from build123d import *

# Parameters (mm, degrees)
SKETCH1_W                  = 5
SKETCH1_H                  = 7
BOSS_EXTRUDE1_DEPTH        = 2.5
SKETCH2_R                  = 0.75
CUT_EXTRUDE1_DEPTH         = 6.5
SKETCH4_R                  = 0.375
CHAMFER1_SIZE              = 0.1
SKETCH5_W                  = 0.8
SKETCH5_H                  = 0.1
CUT_EXTRUDE2_DEPTH         = 10.09068901
LPATTERN1_COUNT            = 2
LPATTERN1_PITCH            = 2.5
LPATTERN2_COUNT            = 2
LPATTERN2_PITCH            = 2.5
CHAMFER1_OF_LPATTERN2_SIZE = 0.1


with BuildPart() as part:
    # Sketch1 → Boss-Extrude1 (new body)
    with BuildSketch(Plane(origin=(0, 0, 0), x_dir=(1, 0, 0), z_dir=(0, 1, 0))):
        Rectangle(SKETCH1_W, SKETCH1_H)
    extrude(amount=BOSS_EXTRUDE1_DEPTH)

    # Sketch2 → Cut-Extrude1 (cut)
    with BuildSketch(Plane(origin=(0, 0, -3.5), x_dir=(-1, 0, 0), z_dir=(0, 0, -1))):
        with Locations((-1.2, 1.25)):
            Circle(SKETCH2_R)
    cut_extrude1 = extrude(amount=-CUT_EXTRUDE1_DEPTH, mode=Mode.SUBTRACT)

    # Sweep1: sweep along a path in Sketch3
    with BuildLine(Plane(origin=(1.2, 0, 0), x_dir=(0, 0, -1), z_dir=(1, 0, 0))) as sweep1_path:
        Line((-3.5, 1.254208417), (-3.8, 1.254208417))
        ThreePointArc((-3.8, 1.254208417), (-4.294974747, 1.049183164), (-4.5, 0.554208417))
        Line((-4.5, 0.554208417), (-4.5, -0.992950224))
    # Sketch4 → Sweep1 (sweep)
    with BuildSketch(Plane.XY.offset(3.5)):
        with Locations((1.2, 1.254208417)):
            Circle(SKETCH4_R)
    sweep1 = sweep(path=sweep1_path.line)

    # Chamfer1
    chamfer1_edges = [part.edges().sort_by_distance(p)[0] for p in [
        (0.825, 1.254208417, 3.5),
        (0.825, -0.992950224, 4.5),
    ]]
    chamfer(chamfer1_edges, length=CHAMFER1_SIZE)

    # Sketch5 → Cut-Extrude2 (cut, through all)
    with BuildSketch(Plane(origin=(0, 0, -3.5), x_dir=(-1, 0, 0), z_dir=(0, 0, -1))):
        with Locations((0, 2.45)):
            Rectangle(SKETCH5_W, SKETCH5_H)
    cut_extrude2 = extrude(amount=-CUT_EXTRUDE2_DEPTH, mode=Mode.SUBTRACT)

    # Mirror6: Cut-Extrude2 across plane
    add(cut_extrude2.mirror(Plane(origin=(0, 1.25, 0), x_dir=(0, 0, 1), z_dir=(0, -1, 0))), mode=Mode.SUBTRACT)

    # LPattern1: Cut-Extrude1 ×2
    with Locations(*[(-i * LPATTERN1_PITCH, 0, 0) for i in range(1, LPATTERN1_COUNT)]):
        add(cut_extrude1, mode=Mode.SUBTRACT)

    # LPattern2: Sweep1 ×2
    with Locations(*[(-i * LPATTERN2_PITCH, 0, 0) for i in range(1, LPATTERN2_COUNT)]):
        add(sweep1)

    # Chamfer1 of LPattern2
    chamfer1_of_lpattern2_edges = [part.edges().sort_by_distance(p)[0] for p in [
        (-1.675, 1.254208417, 3.5),
        (-1.675, -0.992950224, 4.5),
    ]]
    chamfer(chamfer1_of_lpattern2_edges, length=CHAMFER1_OF_LPATTERN2_SIZE)


solid = part.part
Here's how the part is built. I have some questions about the finished solid (model axes, mm). A direction names the side the tool comes from. Round coordinates to 2 decimals unless told otherwise and drop trailing zeros. Loops run counter-clockwise (first coordinate to the right, second up) from the corner with the lowest first, then second, coordinate; pieces in that order, holes last.
1. We'd pull the mould along X, two halves only. Please class faces 4 (the face through (2.5, 1, 0)), 5 (the face through (-1, 2.5, 0)), 6 (the face through (1, 1, 3)): +X half, -X half, draft (parallel to the pull), parting line (faces both ways), or undercut.
Answer list:
face 4: +X half
face 5: draft
face 6: undercut
2. If we section it at A-A on y = 0.4: Write out the boundary of the cut face in (x, z) (3 decimals).
Answer list:
outline: (-2.5, -3.5) - (2.5, -3.5) - (2.5, 3.5) - (-2.5, 3.5) - close; circle Ø0.75 at (-1.3, 4.5); circle Ø0.75 at (1.2, 4.5)
3. If we section it at B-B on z = -0.25: Write out the boundary of the cut face in (x, y).
Answer list:
outline: (-2.5, 0) - (-0.4, 0) - (-0.4, 0.1) - (0.4, 0.1) - (0.4, 0) - (2.5, 0) - (2.5, 2.5) - (0.4, 2.5) - (0.4, 2.4) - (-0.4, 2.4) - (-0.4, 2.5) - (-2.5, 2.5) - close; hole circle Ø1.5 at (-1.3, 1.25); hole circle Ø1.5 at (1.2, 1.25)
4. For P1, Ø1.4, axis at x = -1.3, y = 1.25, coming from the -Z side; P2, Ø0.6, axis at x = 0, z = 0, coming from the +Y side; P3, Ø1.6, axis at x = 1.5, y = 1, coming from the -Z side; P4, Ø0.9, axis at x = 0, z = 1.5, coming from the -Y side, each with a flat end and sliding along its axis, tell me the tip position at first contact or that it passes through.
Answer list:
P1: stops at z = 3
P2: stops at y = 2.4
P3: stops at z = -3.5
P4: stops at y = 0
5. If I drill on line 1 along X through (y, z) = (1.6, -2); line 2 along Y through (x, z) = (1.2, -2); line 3 along X through (y, z) = (0.65, -0.25), over which ranges is the centre line in solid material (lowest first)?
Answer list:
line 1: x = -2.5 to -1.96, -0.64 to 0.54, 1.86 to 2.5
line 2: y = 0 to 0.5, 2 to 2.5
line 3: x = -2.5 to -1.75, -0.85 to 0.75, 1.65 to 2.5
6. Which directions (+Z, -Z, +X, -X, +Y, -Y) give clear straight access to the entire face, cutting with the end or side of a thin tool? Please do faces 1 (the face through (-1.99, 0.96, -0.3)), 2 (the face through (0, 2.4, 0)), 3 (the face through (0, 0.1, 0)).
Answer list:
face 1: -Z
face 2: +Z, -Z, +Y
face 3: +Z, -Z, -Y
7. If we section it at C-C on x = 1.2: Write out the boundary of the cut face in (y, z) (3 decimals), plus the area to 3 significant figures.
Answer list:
outline: (-0.993, 4.225) - (-0.893, 4.125) - (0.554, 4.125) arc R0.325 cw to (0.879, 3.8) - (0.879, 3.6) - (0.779, 3.5) - (0, 3.5) - (0, -3.5) - (0.5, -3.5) - (0.5, 3) - (2, 3) - (2, -3.5) - (2.5, -3.5) - (2.5, 3.5) - (1.729, 3.5) - (1.629, 3.6) - (1.629, 3.8) arc R1.075 ccw to (0.554, 4.875) - (-0.893, 4.875) - (-0.993, 4.775) - close
area: 9.96 mm2
8. If we section it at D-D on z = 3.25: Write out the boundary of the cut face in (x, y).
Answer list:
outline: (-2.5, 0) - (-0.4, 0) - (-0.4, 0.1) - (0.4, 0.1) - (0.4, 0) - (2.5, 0) - (2.5, 2.5) - (0.4, 2.5) - (0.4, 2.4) - (-0.4, 2.4) - (-0.4, 2.5) - (-2.5, 2.5) - close
